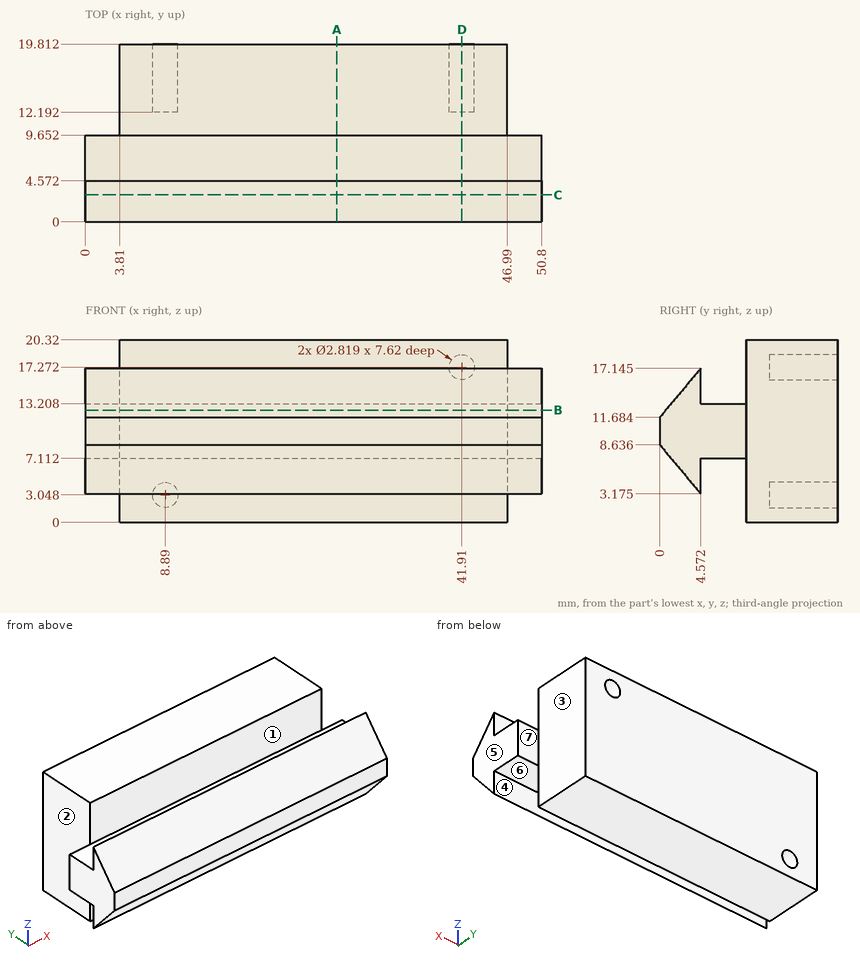
Answer from the drawing. Dimensions are ordinates in mm from the lowest x, y and z of the part. A direction names the side the tool comes from. Coordinates: 2 decimals unless noted, no trailing zeros. Write each loop counter-clockwise with the first axis right and the second up, starting at its lowest first coordinate (ties: lowest second). Pieces come first, ordered by that corner, then holes. Notation, with made-up numbers: (47.25, 38) - (100.25, 38) arc R20 ccw to (100.25, 58) - close; hole circle Ø10 at (-2.5, 81.5). An arc over 180 degrees is marked (long way). Return JSON: item names as keys, results as strings. Group by question number.
Q1. The part is cut by section B-B on z = 12.5. Write down the section's boundary in (x, y).
Q2. The part is cut by section D-D on x = 41.91. Write down the section's boundary in (y, z) (1 decimal).
Q3. Find the intervals of material crossed by line 1 along Z through (x, y) = (41.91, 18); line 2 along Z through (x, y) = (44.5, 5); line 3 along X through (y, z) = (12.75, 4), in increasing order. Write a range as [from, to].
Q4. The part is cut by section A-A on x = 28. Write down the section's boundary in (y, z) (1 decimal).
Q5. The part is cut by section C-C on y = 3. Write down the section's boundary in (x, z), and give its area (3 significant figures).
Q6. Flat-ended cylindrical pins translate along their axes: pin 1 Ø3 at (x, z) = (42, 17) entering from +Y; pin 2 Ø4 at (x, y) = (22.5, 7.5) entering from -Z; pin 3 Ø1.1 at (x, z) = (50, 11.5) entering from +Y; pin 4 Ø2.5 at (x, z) = (8.89, 3.048) entering from -Y. Find the tip coordinate at first contact, or state that the pin passes through.
Q7. Which of the six approach directions +Z, -Z, +X, -X, +Y, -Y give full straight-line access (tool end or side, diameter ignored) to the marked faces 1, 2, 3 and 4?
Q8. For a pull along Y with two mould halves and no side action, classify the marked faces 5, 6 and 7 as +Y half, -Y half, draft (parallel to the pull), parting line (faces both ways), or undercut.
Evaluation:
{
 "1": {"outline": "(0, 0.68) - (50.8, 0.68) - (50.8, 9.65) - (46.99, 9.65) - (46.99, 19.81) - (3.81, 19.81) - (3.81, 9.65) - (0, 9.65) - close"},
 "2": {"outline": "(0, 8.6) - (4.6, 3.2) - (4.6, 7.1) - (9.7, 7.1) - (9.7, 0) - (19.8, 0) - (19.8, 15.9) - (12.2, 15.9) - (12.2, 18.7) - (19.8, 18.7) - (19.8, 20.3) - (9.7, 20.3) - (9.7, 13.2) - (4.6, 13.2) - (4.6, 17.1) - (0, 11.7) - close"},
 "3": {"line 1": "z = [0, 15.86], [18.68, 20.32]", "line 2": "z = [7.11, 13.21]", "line 3": "x = [3.81, 7.85], [9.93, 46.99]"},
 "4": {"outline": "(0, 8.6) - (4.6, 3.2) - (4.6, 7.1) - (9.7, 7.1) - (9.7, 0) - (19.8, 0) - (19.8, 20.3) - (9.7, 20.3) - (9.7, 13.2) - (4.6, 13.2) - (4.6, 17.1) - (0, 11.7) - close"},
 "5": {"outline": "(0, 5.05) - (50.8, 5.05) - (50.8, 15.27) - (0, 15.27) - close", "area": "519 mm2"},
 "6": {"pin 1": "stops at y = 19.81", "pin 2": "stops at z = 7.11", "pin 3": "stops at y = 9.65", "pin 4": "stops at y = 3.63"},
 "7": {"face 1": "+Z, +X, -X", "face 2": "+Z, -Z, -X, +Y", "face 3": "+Z, -Z, +X, +Y", "face 4": "-Z, +X, -X"},
 "8": {"face 5": "draft", "face 6": "undercut", "face 7": "+Y half"}
}
